from build123d import *

# Parameters (mm, degrees)
SKETCH023_R     = 1.7
PAD004_DEPTH    = 2
PAD005_DEPTH    = 2
SKETCH025_W     = 40
SKETCH025_H     = 3
PAD006_DEPTH    = 25
PAD007_DEPTH    = 5
SKETCH027_R     = 1.7
POCKET018_DEPTH = 10


with BuildPart() as part:
    # Sketch023 → Pad004 (new body)
    with BuildSketch(Plane.XY):
        with BuildLine():
            Line((-52.5, 0), (-30.5, 0))
            Line((-30.5, 0), (30.5, 0))
            Line((30.5, 0), (52.5, 0))
            Line((52.5, 0), (52.5, 76.5))
            ThreePointArc((52.5, 76.5), (49.886128, 88.747449), (42.5, 98.86068))
            Line((42.5, 98.86068), (30, 110.04102))
            ThreePointArc((30, 110.04102), (0, 121.5), (-30, 110.04102))
            Line((-30, 110.04102), (-42.5, 98.86068))
            ThreePointArc((-42.5, 98.86068), (-49.886128, 88.747449), (-52.5, 76.5))
            Line((-52.5, 76.5), (-52.5, 0))
        make_face()
        with Locations((17.511522, 32.982072)):
            Circle(SKETCH023_R, mode=Mode.SUBTRACT)
        with Locations((17.511522, 47.982072)):
            Circle(SKETCH023_R, mode=Mode.SUBTRACT)
        with Locations((32.511522, 47.982072)):
            Circle(SKETCH023_R, mode=Mode.SUBTRACT)
        with Locations((32.511522, 32.982072)):
            Circle(SKETCH023_R, mode=Mode.SUBTRACT)
        with Locations((-7.5, 32.982072)):
            Circle(SKETCH023_R, mode=Mode.SUBTRACT)
        with Locations((-7.5, 47.982072)):
            Circle(SKETCH023_R, mode=Mode.SUBTRACT)
        with Locations((7.5, 47.982072)):
            Circle(SKETCH023_R, mode=Mode.SUBTRACT)
        with Locations((7.5, 32.982072)):
            Circle(SKETCH023_R, mode=Mode.SUBTRACT)
        with Locations((-32.511522, 32.982072)):
            Circle(SKETCH023_R, mode=Mode.SUBTRACT)
        with Locations((-32.511522, 47.982072)):
            Circle(SKETCH023_R, mode=Mode.SUBTRACT)
        with Locations((-17.511522, 47.982072)):
            Circle(SKETCH023_R, mode=Mode.SUBTRACT)
        with Locations((-17.511522, 32.982072)):
            Circle(SKETCH023_R, mode=Mode.SUBTRACT)
        with Locations((17.511522, 57.993594)):
            Circle(SKETCH023_R, mode=Mode.SUBTRACT)
        with Locations((17.511522, 72.993594)):
            Circle(SKETCH023_R, mode=Mode.SUBTRACT)
        with Locations((32.511522, 72.993594)):
            Circle(SKETCH023_R, mode=Mode.SUBTRACT)
        with Locations((32.511522, 57.993594)):
            Circle(SKETCH023_R, mode=Mode.SUBTRACT)
        with Locations((-7.5, 57.993594)):
            Circle(SKETCH023_R, mode=Mode.SUBTRACT)
        with Locations((-7.5, 72.993594)):
            Circle(SKETCH023_R, mode=Mode.SUBTRACT)
        with Locations((7.5, 72.993594)):
            Circle(SKETCH023_R, mode=Mode.SUBTRACT)
        with Locations((7.5, 57.993594)):
            Circle(SKETCH023_R, mode=Mode.SUBTRACT)
        with Locations((-32.511522, 57.993594)):
            Circle(SKETCH023_R, mode=Mode.SUBTRACT)
        with Locations((-32.511522, 72.993594)):
            Circle(SKETCH023_R, mode=Mode.SUBTRACT)
        with Locations((-17.511522, 72.993594)):
            Circle(SKETCH023_R, mode=Mode.SUBTRACT)
        with Locations((-17.511522, 57.993594)):
            Circle(SKETCH023_R, mode=Mode.SUBTRACT)
        with Locations((17.511522, 83.005116)):
            Circle(SKETCH023_R, mode=Mode.SUBTRACT)
        with Locations((17.511522, 98.005116)):
            Circle(SKETCH023_R, mode=Mode.SUBTRACT)
        with Locations((32.511522, 98.005116)):
            Circle(SKETCH023_R, mode=Mode.SUBTRACT)
        with Locations((32.511522, 83.005116)):
            Circle(SKETCH023_R, mode=Mode.SUBTRACT)
        with Locations((-7.5, 83.005116)):
            Circle(SKETCH023_R, mode=Mode.SUBTRACT)
        with Locations((-7.5, 98.005116)):
            Circle(SKETCH023_R, mode=Mode.SUBTRACT)
        with Locations((7.5, 98.005116)):
            Circle(SKETCH023_R, mode=Mode.SUBTRACT)
        with Locations((7.5, 83.005116)):
            Circle(SKETCH023_R, mode=Mode.SUBTRACT)
        with Locations((-32.511522, 83.005116)):
            Circle(SKETCH023_R, mode=Mode.SUBTRACT)
        with Locations((-32.511522, 98.005116)):
            Circle(SKETCH023_R, mode=Mode.SUBTRACT)
        with Locations((-17.511522, 98.005116)):
            Circle(SKETCH023_R, mode=Mode.SUBTRACT)
        with Locations((-17.511522, 83.005116)):
            Circle(SKETCH023_R, mode=Mode.SUBTRACT)
        with Locations((-7.5, 90.505116)):
            Circle(SKETCH023_R, mode=Mode.SUBTRACT)
        with Locations((-7.5, 105.505116)):
            Circle(SKETCH023_R, mode=Mode.SUBTRACT)
        with Locations((7.5, 105.505116)):
            Circle(SKETCH023_R, mode=Mode.SUBTRACT)
        with Locations((7.5, 90.505116)):
            Circle(SKETCH023_R, mode=Mode.SUBTRACT)
        with Locations((-24.827374, 3)):
            Circle(SKETCH023_R, mode=Mode.SUBTRACT)
        with Locations((-7.5, 3)):
            Circle(SKETCH023_R, mode=Mode.SUBTRACT)
        with Locations((7.5, 3)):
            Circle(SKETCH023_R, mode=Mode.SUBTRACT)
        with Locations((25.172626, 3)):
            Circle(SKETCH023_R, mode=Mode.SUBTRACT)
    extrude(amount=PAD004_DEPTH)

    # Sketch024 (on Face56 of Pad004) → Pad005 (join)
    with BuildSketch(Plane.XY.offset(2)):
        with BuildLine():
            Line((-52.5, 0), (-30.5, 0))
            Line((-30.5, 0), (-30.5, 6.5))
            Line((-30.5, 6.5), (30.5, 6.5))
            Line((30.5, 6.5), (30.5, 0))
            Line((30.5, 0), (52.5, 0))
            Line((52.5, 0), (52.5, 76.5))
            ThreePointArc((52.5, 76.5), (49.886128, 88.747449), (42.5, 98.86068))
            Line((42.5, 98.86068), (30, 110.04102))
            ThreePointArc((30, 110.04102), (0, 121.5), (-30, 110.04102))
            Line((-30, 110.04102), (-42.5, 98.86068))
            ThreePointArc((-42.5, 98.86068), (-49.886128, 88.747449), (-52.5, 76.5))
            Line((-52.5, 76.5), (-52.5, 0))
        make_face()
        with BuildLine():
            Line((-50.5, 2), (-50.5, 76.5))
            ThreePointArc((-40.126205, 98.86068), (-47.780263, 88.82493), (-50.5, 76.5))
            Line((-40.126205, 98.86068), (-26.907285, 110.04102))
            ThreePointArc((26.907285, 110.04102), (0, 119.500023), (-26.907285, 110.04102))
            Line((26.907285, 110.04102), (40.126205, 98.86068))
            ThreePointArc((50.5, 76.5), (47.780263, 88.82493), (40.126205, 98.86068))
            Line((50.5, 76.5), (50.5, 2.779082))
            Line((50.5, 2.779082), (35.5, 2.779082))
            ThreePointArc((32.5, 5.779082), (33.37868, 3.657761), (35.5, 2.779082))
            Line((32.5, 5.779082), (32.5, 9.5))
            Line((32.5, 9.5), (-32.5, 9.5))
            Line((-32.5, 9.5), (-32.5, 5))
            ThreePointArc((-35.5, 2), (-33.37868, 2.87868), (-32.5, 5))
            Line((-35.5, 2), (-50.5, 2))
        make_face(mode=Mode.SUBTRACT)
    extrude(amount=PAD005_DEPTH)

    # Sketch025 (on Face60 of Pad005) → Pad006 (join)
    with BuildSketch(Plane.XY.offset(4)):
        with BuildLine():
            Line((-52.5, 0), (-30.5, 0))
            Line((-30.5, 0), (-30.5, 6.5))
            Line((-32.5, 9.5), (-30.5, 6.5))
            Line((-32.5, 9.5), (-32.5, 5))
            ThreePointArc((-35.5, 2), (-33.37868, 2.87868), (-32.5, 5))
            Line((-35.5, 2), (-50.5, 2))
            Line((-50.5, 2), (-52.5, 2))
            Line((-52.5, 2), (-52.5, 0))
        make_face()
        with Locations((0, 8)):
            Rectangle(SKETCH025_W, SKETCH025_H)
        with BuildLine():
            Line((30.5, 6.5), (30.5, 0))
            Line((30.5, 0), (52.5, 0))
            Line((52.5, 2.779082), (52.5, 0))
            Line((50.5, 2.779082), (52.5, 2.779082))
            Line((50.5, 2.779082), (35.5, 2.779082))
            ThreePointArc((32.5, 5.779082), (33.37868, 3.657761), (35.5, 2.779082))
            Line((32.5, 5.779082), (32.5, 9.5))
            Line((30.5, 6.5), (32.5, 9.5))
        make_face()
    extrude(amount=PAD006_DEPTH)

    # Sketch026 (on Face102 of Pad006) → Pad007 (join)
    with BuildSketch(Plane.XY.offset(29)):
        with BuildLine():
            Line((-52.5, 0), (-30.5, 0))
            Line((-30.5, 0), (-30.5, 6.5))
            Line((-30.5, 6.5), (30.5, 6.5))
            Line((30.5, 6.5), (30.5, 0))
            Line((30.5, 0), (52.5, 0))
            Line((52.5, 2.779082), (52.5, 0))
            Line((50.5, 2.779082), (52.5, 2.779082))
            Line((50.5, 2.779082), (35.5, 2.779082))
            ThreePointArc((32.5, 5.779082), (33.37868, 3.657761), (35.5, 2.779082))
            Line((32.5, 5.779082), (32.5, 9.5))
            Line((32.5, 9.5), (-32.5, 9.5))
            Line((-32.5, 9.5), (-32.5, 5))
            ThreePointArc((-35.5, 2), (-33.37868, 2.87868), (-32.5, 5))
            Line((-35.5, 2), (-50.5, 2))
            Line((-52.5, 2), (-50.5, 2))
            Line((-52.5, 0), (-52.5, 2))
        make_face()
    extrude(amount=PAD007_DEPTH)

    # Sketch027 (on Face114 of Pad007) → Pocket018 (cut)
    with BuildSketch(Plane(origin=(0, 9.5, 0), x_dir=(-1, 0, 0), z_dir=(0, 1, 0))):
        with Locations((-14.881968, 23)):
            Circle(SKETCH027_R)
        with Locations((0, 23)):
            Circle(SKETCH027_R)
        with Locations((15.118032, 23)):
            Circle(SKETCH027_R)
        with Locations((15.118032, 7)):
            Circle(SKETCH027_R)
        with Locations((0, 7)):
            Circle(SKETCH027_R)
        with Locations((-14.881968, 7)):
            Circle(SKETCH027_R)
    extrude(amount=-POCKET018_DEPTH, mode=Mode.SUBTRACT)


solid = part.part
Source: CAD feature listing. Evaluate the final solid. Frame: model axes, mm. A direction names the side the tool comes from. Coordinates: 2 decimals unless noted, no trailing zeros. Order: outer loops, then holes, each group sorted by start corner. A loop starts at its lowest first (then second) coordinate and runs counter-clockwise, first axis right, second up. Notation, with made-up numbers: M 83,-32 L 95,-32 A38 cw 95,7 Z; hole C 42.25,-24.5 d5. An arc over 180 degrees is marked long. Write each question's results on one line, items separated by ' | '. Start each with the question number.
Item 1: Line query: probe 1 along Z at (x, y) = (0, 8); probe 2 along Z at (x, y) = (27, 76.5); probe 3 along Y at (x, z) = (-14, 18.5). Output: solid intervals per line, ascending.
Item 2: Cut plane B-B (x = -7.5). Count the separate pieces of the cut face and the enclosed holes in it, and give its area (3 significant figures).
Item 3: Cut plane A-A (z = 15). Return loops of the section in (x, y), and give its area (3 significant figures).
Item 4: Draft query along Z for faces 1 (the face through (-31.7, 71.5, 1)), 2 (the face through (0.37, 8.02, 5.34)), 3 (the face through (-15.9, 8.02, 5.49)). Return one class per face: pulls with the +Z half, pulls with the -Z half, needs draft (parallel to the pull), parting line crosses it, or undercut.
Item 5: Set-up query: faces 4 (the face through (-36.16, 104.53, 1.97)), 5 (the face through (-47.7, 89, 3)). Return all of +Z, -Z, +X, -X, +Y, -Y with unobstructed straight access to the full face (end or side cutting, diameter ignored); none if empty.
Item 6: First-contact query: pin 1 Ø8 at (x, z) = (17, 24.5) entering from -Y; pin 2 Ø5 at (x, z) = (-19, 7.5) entering from +Y; pin 3 Ø6 at (x, y) = (-35, 65.5) entering from +Z. Flat tips, straight axial feed; report the tip coordinate or a pass-through.
Checked values:
1) probe 1: z = 0 to 5.3, 8.7 to 21.3, 24.7 to 34 | probe 2: z = 0 to 2 | probe 3: y = 6.5 to 9.5
2) separate pieces: 10 | enclosed holes: 0 | area: 281 mm2
3) outline: M -52.5,0 L -30.5,0 L -30.5,6.5 L -32.5,9.5 L -32.5,5 A3 cw -35.5,2 L -52.5,2 Z; M -20,6.5 L 20,6.5 L 20,9.5 L -20,9.5 Z; M 30.5,0 L 52.5,0 L 52.5,2.78 L 35.5,2.78 A3 cw 32.5,5.78 L 32.5,9.5 L 30.5,6.5 Z | area: 251 mm2
4) face 1: needs draft | face 2: undercut | face 3: undercut
5) face 4: +Z, -Z, -X, +Y | face 5: +Z
6) pin 1: stops at y = 6.5 | pin 2: stops at y = 9.5 | pin 3: stops at z = 2
